```python
from build123d import *

# Parameters (mm, degrees)
SKETCH_R      = 49
PAD_DEPTH     = 5.8
SKETCH001_R   = 3.75
SKETCH001_R_2 = 1.5
SKETCH001_R_3 = 1.75
POCKET_DEPTH  = 5.801


with BuildPart() as part:
    # Sketch → Pad (new body)
    with BuildSketch(Plane.XY):
        Circle(SKETCH_R)
    extrude(amount=PAD_DEPTH)

    # Sketch001 (on Face3 of Pad) → Pocket (cut, through all)
    with BuildSketch(Plane.XY.offset(5.8)):
        with Locations((0, 31.75)):
            Circle(SKETCH001_R)
        with Locations((0, -31.75)):
            Circle(SKETCH001_R)
        with Locations((-17.5, 0)):
            Circle(SKETCH001_R)
        with Locations((17.5, 0)):
            Circle(SKETCH001_R)
        with Locations((23.098822, 23.098822)):
            Circle(SKETCH001_R_2)
        with Locations((23.098822, -23.098822)):
            Circle(SKETCH001_R_2)
        with Locations((30.696626, 11.172658)):
            Circle(SKETCH001_R_3)
        with Locations((30.696626, -11.172658)):
            Circle(SKETCH001_R_3)
    extrude(amount=-POCKET_DEPTH, mode=Mode.SUBTRACT)


solid = part.part
```
Could you check a few things on this model? Use its own coordinates, in mm. Round coordinates to 2 decimals unless told otherwise and drop trailing zeros. Loops run counter-clockwise (first coordinate to the right, second up) from the corner with the lowest first, then second, coordinate; pieces in that order, holes last.
Q1. I want a section at A-A (y = 0). Write out the boundary of the cut face in (x, z), and give its area (3 significant figures).
Q2. I want a section at D-D (y = -31.75). Write out the boundary of the cut face in (x, z).
Q3. Please list where these lines run through material, in increasing order: L1, parallel to Y at x = 0, z = 2.9; L2, parallel to Y at x = -3, z = 1.4; L3, parallel to X at y = -22, z = 0.8.
Q4. Thinking about a two-plate mould opening in Y: for faces 1 (the cylindrical face through (21.9, 22.2, 2.9)), 2 (the cylindrical face through (0, -28, 3)), 3 (the cylindrical face through (26.34, 41.32, 2.86)), 4 (the flat face through (-1, 1, 5.8)), which applies, pulls with the +Y half, pulls with the -Y half, needs draft (parallel to the pull), parting line crosses it, or undercut?
Q5. I want a section at B-B (x = -17.5). Write out the boundary of the cut face in (y, z), and give its area (3 significant figures).
Q6. I want a section at C-C (z = 3.05). Give the number of separate pieces and of enclosed holes in the cut face, and give its area (3 significant figures).
Answer below:
1. outline: (-49, 0) - (-21.25, 0) - (-21.25, 5.8) - (-49, 5.8) - close; (-13.75, 0) - (13.75, 0) - (13.75, 5.8) - (-13.75, 5.8) - close; (21.25, 0) - (49, 0) - (49, 5.8) - (21.25, 5.8) - close
1. area: 481 mm2
2. outline: (-37.32, 0) - (-3.75, 0) - (-3.75, 5.8) - (-37.32, 5.8) - close; (3.75, 0) - (37.32, 0) - (37.32, 5.8) - (3.75, 5.8) - close
3. L1: y = -49 to -35.5, -28 to 28, 35.5 to 49
3. L2: y = -48.91 to -34, -29.5 to 29.5, 34 to 48.91
3. L3: x = -43.78 to 22.08, 24.12 to 43.78
4. face 1: undercut
4. face 2: undercut
4. face 3: parting line crosses it
4. face 4: needs draft
5. outline: (-45.77, 0) - (-3.75, 0) - (-3.75, 5.8) - (-45.77, 5.8) - close; (3.75, 0) - (45.77, 0) - (45.77, 5.8) - (3.75, 5.8) - close
5. area: 487 mm2
6. separate pieces: 1
6. enclosed holes: 8
6. area: 7,330 mm2
